Part model, mm, in its own coordinate system. A direction names the side the tool comes from. Give positions to 0.01 mm unless a question says otherwise; leave off trailing zeros. Order: outer loops, then holes, each group sorted by start corner. A loop starts at its lowest first (then second) coordinate and runs counter-clockwise, first axis right, second up. Notation, with made-up numbers: (5.5, 88) -> (27.5, 88) arc R22 ccw to (27.5, 110) -> close; hole circle Ø2 at (36, -35). An arc over 180 degrees is marked (long way). Write item = value, one per line. Start each with the question number.
Item 1: Drill centre lines: line 1 along Z through (x, y) = (7, 6.5); line 2 along Y through (x, z) = (4, 8.75); line 3 along Y through (x, z) = (15, 0.5). Where is each one in solid material? Low to high.
Item 2: Tool access for faces 1 (the face through (10, 14, 6)), 2 (the face through (10, 15, 6)): list every direction of +Z, -Z, +X, -X, +Y, -Y with a clear straight run to the whole face (end or side of a thin tool).
Item 3: Band-saw the part on A-A on x = 6.75. Write the cut outline in (y, z).
Item 4: Band-saw the part on C-C on z = 4. Write the cut outline in (x, y), plus the area to 3 significant figures.
Item 5: Flat gauge pins, fed straight in: P1, Ø1.5, axis at x = 8.5, z = 2.5, coming from the -Y side; P2, Ø3, axis at x = 5.5, z = 2.5, coming from the -Y side; P3, Ø3.5, axis at x = 8, y = 8.5, coming from the +Z side. Where does each tip first touch, or does it go through?
Item 6: Band-saw the part on B-B on y = 4. Write the cut outline in (x, z).
```python
from build123d import *

# Parameters (mm, degrees)
SKETCH_1_W            = 20
SKETCH_1_H            = 10
BASEPLATE_DEPTH       = 1
EDGEFLANGE_DEPTH      = 20
EDGEFLANGE_FLAT_DEPTH = 1


# Sheet-metal steps are written as plain solids
with BuildPart() as part:
    # BasePlate: sheet metal written as solids
    # Sketch 1 → BasePlate (new body)
    with BuildSketch(Plane.XY):
        with Locations((10, 5)):
            Rectangle(SKETCH_1_W, SKETCH_1_H)
    extrude(amount=-BASEPLATE_DEPTH)

    # EdgeFlange: sheet metal written as solids
    # EdgeFlange bend section (on a plane across the edge) → EdgeFlange (add)
    with BuildSketch(Plane(origin=(20, 15, 0), x_dir=(0, -1, 0), z_dir=(-1, 0, 0))):
        with BuildLine():
            Line((0, 2), (1, 2))
            ThreePointArc((1, 2), (1.585786438, 0.585786438), (3, 0))
            Line((3, 0), (5, 0))
            Line((5, 0), (5, -1))
            Line((5, -1), (3, -1))
            ThreePointArc((3, -1), (0.878679656, -0.121320344), (0, 2))
        make_face()
    extrude(amount=EDGEFLANGE_DEPTH)

    # EdgeFlange profile (on flange) → EdgeFlange flat (add)
    with BuildSketch(Plane(origin=(0, 15, 0), x_dir=(-1, 0, 0), z_dir=(0, 1, 0))):
        Polygon((-20, 10), (-20, 2), (0, 2), (0, 10), (-2, 10), (-18, 10), align=None)
    extrude(amount=-EDGEFLANGE_FLAT_DEPTH)


solid = part.part
```
Values found:
q1.line_1 = -1 to 0
q1.line_2 = 14 to 15
q1.line_3 = 13.32 to 14.6
q2.face_1 = +Z, +X, -X, -Y
q2.face_2 = +Z, -Z, +X, -X, +Y
q3.outline = (0, -1) -> (12, -1) arc R3 ccw to (15, 2) -> (15, 10) -> (14, 10) -> (14, 2) arc R2 cw to (12, 0) -> (0, 0) -> close
q4.outline = (0, 14) -> (20, 14) -> (20, 15) -> (0, 15) -> close
q4.area = 20.0 mm^2
q5.P1 = 13.98
q5.P2 = 13.73
q5.P3 = 0
q6.outline = (0, -1) -> (20, -1) -> (20, 0) -> (0, 0) -> close
